```python
from build123d import *

# Parameters (mm, degrees)
F4_DEPTH = 6.35


# Not quite as in the source:
# - the program builds the solid bodies; features that only make, move or delete a surface that nothing else refers to are left out


with BuildPart() as f2:
    # F0 (on Front) → F2 (revolve)
    with BuildSketch(Plane.XZ):
        with BuildLine():
            ThreePointArc((24.3612137616, 20.3615756773), (15.8531486732, 27.508910868), (5.403325821, 31.2868434022))
            ThreePointArc((5.403325821, 31.2868434022), (2.7115698388, 31.6339989412), (0, 31.75))
            Line((0, 31.75), (0, -31.75))
            ThreePointArc((0, -31.75), (2.736702771, -31.6318345649), (5.4530349168, -31.2782178232))
            ThreePointArc((5.4530349168, -31.2782178232), (15.8968413055, -27.483684915), (24.39353828, -20.322839127))
            ThreePointArc((24.39353828, -20.322839127), (27.508910868, -15.8531486732), (29.8142486784, -10.9166421459))
            ThreePointArc((29.8142486784, -10.9166421459), (31.2623167371, -5.5434693316), (31.75, 0))
            ThreePointArc((31.75, 0), (31.2579024825, 5.5683060617), (29.796864101, 10.9640042752))
            ThreePointArc((29.796864101, 10.9640042752), (27.483684915, 15.8968413055), (24.3612137616, 20.3615756773))
        make_face()
    revolve(axis=Axis((0, 0, 0), (0, 0, -1)))

    # F3 (on Front) → F4 (join, symmetric)
    with BuildSketch(Plane.XZ):
        with BuildLine():
            Line((5.376374884, 38.1001170391), (5.3115624093, 54.484895228))
            ThreePointArc((5.3115624093, 54.484895228), (-0.1171664817, 54.7430614347), (-5.5447405359, 54.4616595011))
            Line((-5.5447405359, 54.4616595011), (-5.5087377694, 45.3600575994))
            Line((-5.5087377694, 45.3600575994), (-19.2836534145, 45.3600575994))
            Line((-19.2836534145, 45.3600575994), (-19.2836534145, 38.1001170391))
            Line((-19.2836534145, 38.1001170391), (-5.4800199737, 38.1001170391))
            Line((-5.4800199737, 38.1001170391), (-5.4530349168, 31.2782178232))
            Line((-5.4530349168, 31.2782178232), (-5.4530349168, 22.3882178232))
            Line((-5.4530349168, 22.3882178232), (5.403325821, 22.3882178232))
            Line((5.403325821, 22.3882178232), (5.403325821, 31.2868434022))
            Line((5.403325821, 31.2868434022), (5.376374884, 38.1001170391))
        make_face()
        with BuildLine():
            Line((22.0904282909, 6.5146914857), (29.796864101, 10.9640042752))
            Line((29.796864101, 10.9640042752), (49.8410845946, 22.6424996338))
            ThreePointArc((49.8410845946, 22.6424996338), (47.3502986425, 27.472999867), (44.3928103923, 32.0327159121))
            Line((44.3928103923, 32.0327159121), (36.5285933135, 27.4507356508))
            Line((36.5285933135, 27.4507356508), (29.6411354909, 39.3801625345))
            Line((29.6411354909, 39.3801625345), (23.3538425357, 35.7501922543))
            Line((23.3538425357, 35.7501922543), (30.2556592562, 23.79589503))
            Line((30.2556592562, 23.79589503), (24.3612137616, 20.3615756773))
            Line((24.3612137616, 20.3615756773), (16.6622479219, 15.9165756773))
            Line((16.6622479219, 15.9165756773), (22.0904282909, 6.5146914857))
        make_face()
        with BuildLine():
            Line((16.6871024699, -15.8735263375), (24.39353828, -20.322839127))
            Line((24.39353828, -20.322839127), (30.307481801, -23.7061357493))
            Line((30.307481801, -23.7061357493), (44.5295221853, -31.8423955942))
            ThreePointArc((44.5295221853, -31.8423955942), (47.4674651242, -27.2700615677), (49.9375509282, -22.4289435891))
            Line((49.9375509282, -22.4289435891), (42.0373310829, -17.9093219486))
            Line((42.0373310829, -17.9093219486), (48.9247889055, -5.9798950649))
            Line((48.9247889055, -5.9798950649), (42.6374959503, -2.3499247848))
            Line((42.6374959503, -2.3499247848), (35.7356792298, -14.3042220091))
            Line((35.7356792298, -14.3042220091), (29.8142486784, -10.9166421459))
            Line((29.8142486784, -10.9166421459), (22.1152828388, -6.4716421459))
            Line((22.1152828388, -6.4716421459), (16.6871024699, -15.8735263375))
        make_face()
        with BuildLine():
            Line((-5.403325821, -22.3882178232), (-5.403325821, -31.2868434022))
            Line((-5.403325821, -31.2868434022), (-5.3115624093, -54.484895228))
            ThreePointArc((-5.3115624093, -54.484895228), (0.1171664817, -54.7430614347), (5.5447405359, -54.4616595011))
            Line((5.5447405359, -54.4616595011), (5.5087377694, -45.3600575994))
            Line((5.5087377694, -45.3600575994), (19.2836534145, -45.3600575994))
            Line((19.2836534145, -45.3600575994), (19.2836534145, -38.1001170391))
            Line((19.2836534145, -38.1001170391), (5.4800199737, -38.1001170391))
            Line((5.4800199737, -38.1001170391), (5.4530349168, -31.2782178232))
            Line((5.4530349168, -31.2782178232), (5.4530349168, -22.3882178232))
            Line((5.4530349168, -22.3882178232), (-5.403325821, -22.3882178232))
        make_face()
        with BuildLine():
            Line((-29.796864101, -10.9640042752), (-49.8410845946, -22.6424996338))
            ThreePointArc((-49.8410845946, -22.6424996338), (-47.3502986425, -27.472999867), (-44.3928103923, -32.0327159121))
            Line((-44.3928103923, -32.0327159121), (-36.5285933135, -27.4507356508))
            Line((-36.5285933135, -27.4507356508), (-29.6411354909, -39.3801625345))
            Line((-29.6411354909, -39.3801625345), (-23.3538425357, -35.7501922543))
            Line((-23.3538425357, -35.7501922543), (-30.2556592562, -23.79589503))
            Line((-30.2556592562, -23.79589503), (-24.3612137616, -20.3615756773))
            Line((-24.3612137616, -20.3615756773), (-16.6622479219, -15.9165756773))
            Line((-16.6622479219, -15.9165756773), (-22.0904282909, -6.5146914857))
            Line((-22.0904282909, -6.5146914857), (-29.796864101, -10.9640042752))
        make_face()
        with BuildLine():
            Line((-16.6871024699, 15.8735263375), (-24.39353828, 20.322839127))
            Line((-24.39353828, 20.322839127), (-30.307481801, 23.7061357493))
            Line((-30.307481801, 23.7061357493), (-44.5295221853, 31.8423955942))
            ThreePointArc((-44.5295221853, 31.8423955942), (-47.4674651242, 27.2700615677), (-49.9375509282, 22.4289435891))
            Line((-49.9375509282, 22.4289435891), (-42.0373310829, 17.9093219486))
            Line((-42.0373310829, 17.9093219486), (-48.9247889055, 5.9798950649))
            Line((-48.9247889055, 5.9798950649), (-42.6374959503, 2.3499247848))
            Line((-42.6374959503, 2.3499247848), (-35.7356792298, 14.3042220091))
            Line((-35.7356792298, 14.3042220091), (-29.8142486784, 10.9166421459))
            Line((-29.8142486784, 10.9166421459), (-22.1152828388, 6.4716421459))
            Line((-22.1152828388, 6.4716421459), (-16.6871024699, 15.8735263375))
        make_face()
    extrude(amount=F4_DEPTH, both=True)


solid = f2.part
```
Verification items for the finished model (mm, model axes). A direction names the side the tool comes from. Round coordinates to 2 decimals unless told otherwise and drop trailing zeros. Order: outer loops, then holes, each group sorted by start corner. A loop starts at its lowest first (then second) coordinate and runs counter-clockwise, first axis right, second up. Notation, with made-up numbers: (3, 81.5) - (50, 81.5) arc R38 ccw to (50, 119.5) - close; hole circle Ø11 at (23.25, 2.25). An arc over 180 degrees is marked (long way). Use CSV: the item, a comma, the result in double quotes.
(1) Section check A-A on x = -38. Record the boundary of the cut face in (y, z).
Entries:
outline,"(-6.35, -28.31) - (6.35, -28.31) - (6.35, -15.74) - (-6.35, -15.74) - close; (-6.35, 10.38) - (6.35, 10.38) - (6.35, 28.11) - (-6.35, 28.11) - close"
(2) Thickness scan on probe 1 along Y at (x, z) = (-34, -28.5); probe 2 along X at (y, z) = (3, 4); probe 3 along Z at (x, y) = (19, 5.5). Record the ranges inside material, lowest first. Write a range as from..to.
Entries:
probe 1,"-6.35..6.35"
probe 2,"-45.5..-41.68, -31.35..31.35"
probe 3,"-45.36..-38.1, -24.84..24.84"
(3) Section check C-C on y = -19. Record the boundary of the cut face in (x, z).
Entries:
outline,"circle Ø50.87 at (0, 0)"
(4) Access from +Z, -Z, +X, -X, +Y, -Y to the whole of each face (thin tool, end or side, straight path). Record for faces 1 (the face through (26.756, 0.089, 29.857)), 2 (the face through (45.43, 0.09, -12.03)), 3 (the face through (-45.43, -0.09, 12.03)).
Entries:
face 1,"+Y, -Y"
face 2,"+X, +Y, -Y"
face 3,"-X, +Y, -Y"
(5) Mould release check, pull along X, two halves, no side actions. Record for faces 4 (the face through (-32.816, -0.089, 12.634)), 5 (the face through (33.133, 0.089, 33.332)), 6 (the face through (-12, 0, 45.36)), 7 (the face through (19.284, 0, -42)): released by +X, released by -X, zero draft, split by the parting line, or undercut.
Entries:
face 4,"undercut"
face 5,"undercut"
face 6,"zero draft"
face 7,"released by +X"
(6) Section check D-D on x = -22. Record the boundary of the cut face in (y, z), and give its area (3 significant figures).
Entries:
outline,"circle Ø45.78 at (0, 0)"
area,"1,650 mm^2"
(7) Section check B-B on z = -34. Record the boundary of the cut face in (x, y).
Entries:
outline,"(-32.75, -6.35) - (-24.36, -6.35) - (-24.36, 6.35) - (-32.75, 6.35) - close; (-5.39, -6.35) - (5.46, -6.35) - (5.46, 6.35) - (-5.39, 6.35) - close"
(8) Gauge pin test, flat ends, axial feed: pin 1 Ø1.5 at (y, z) = (-1, 25.5) entering from +X; pin 2 Ø4 at (x, y) = (-9.5, -2) entering from +Z; pin 3 Ø21 at (x, z) = (-41, 14) entering from -Y. Record the tip position at first contact, or that the pin passes through.
Entries:
pin 1,"x = 48.83"
pin 2,"z = 45.36"
pin 3,"y = -6.35"
